```python
from build123d import *

# Parameters (mm, degrees)
SKETCH1_W               = 520
SKETCH1_H               = 75
SKETCH1_W_2             = 440
SKETCH1_H_2             = 60
BOSS_EXTRUDE1_DEPTH     = 10
BOSS_EXTRUDE2_DEPTH     = 575
SKETCH3_W               = 520
SKETCH3_H               = 75
BOSS_EXTRUDE3_DEPTH     = 35
CHAMFER1_SIZE           = 19
CHAMFER1_SIZE_2         = 10.969655115
FILLET1_R               = 30
SKETCH4_R               = 7.5
BOSS_EXTRUDE4_DEPTH     = 20
BOSS_EXTRUDE5_START     = 20
SKETCH5_R               = 7.5
BOSS_EXTRUDE5_DEPTH     = 20
SKETCH6_R               = 15
BOSS_EXTRUDE6_DEPTH     = 30
BOSS_EXTRUDE7_START     = 30
SKETCH7_R               = 15
BOSS_EXTRUDE7_DEPTH     = 30
CUT_EXTRUDE1_DEPTH      = 250
CUT_EXTRUDE1_DEPTH_BACK = 250
SKETCH8_R               = 16.5


with BuildPart() as part:
    # Sketch1 → Boss-Extrude1 (new body)
    with BuildSketch(Plane(origin=(0, 0, 0), x_dir=(0, 0, -1), z_dir=(1, 0, 0))):
        with Locations((0, 37.5)):
            Rectangle(SKETCH1_W, SKETCH1_H)
        with Locations((0, 34)):
            Rectangle(SKETCH1_W_2, SKETCH1_H_2, mode=Mode.SUBTRACT)
    extrude(amount=-BOSS_EXTRUDE1_DEPTH)

    # Sketch2 → Boss-Extrude2 (add)
    with BuildSketch(Plane.ZY.offset(10)):
        Polygon((260, 0), (260, 75), (207, 75), (207, 64), (220, 64), (220, 4), (-220, 4), (-220, 64), (-207, 64), (-207, 75), (-260, 75), (-260, 0), align=None)
    extrude(amount=BOSS_EXTRUDE2_DEPTH)

    # Sketch3 → Boss-Extrude3 (add)
    with BuildSketch(Plane(origin=(0, 0, 0), x_dir=(0, 0, -1), z_dir=(1, 0, 0))):
        with Locations((0, 37.5)):
            Rectangle(SKETCH3_W, SKETCH3_H)
    extrude(amount=BOSS_EXTRUDE3_DEPTH)

    # Chamfer1
    # the kernel refuses this chamfer: 19, 10.969655115 mm, written as the material it takes off along each edge
    with BuildSketch(Plane(origin=(-10, 75, 207), x_dir=(0, 0.01932676561270119, 0.9998132206222079), z_dir=(-1, 0, 0))) as chamfer1_piece_1:
        Polygon((CHAMFER1_SIZE * 0.999813220622, -CHAMFER1_SIZE * 0.0193267656127), (-CHAMFER1_SIZE_2 * 0.019326765612, -CHAMFER1_SIZE_2 * 0.999813220586), (0, 0), align=None)
    extrude(amount=624.154629338, mode=Mode.SUBTRACT)
    with BuildSketch(Plane(origin=(-10, 75, -207), x_dir=(0, 0.057893862402678804, -0.9983227437537922), z_dir=(-1, 0, 0))) as chamfer1_piece_2:
        Polygon((CHAMFER1_SIZE_2 * 0.998322743718, CHAMFER1_SIZE_2 * 0.0578938624006), (-CHAMFER1_SIZE * 0.0578938624027, CHAMFER1_SIZE * 0.998322743754), (0, 0), align=None)
    extrude(amount=624.154629338, mode=Mode.SUBTRACT)

    # Fillet1
    fillet1_edges = [part.edges().sort_by_distance(p)[0] for p in [
        (-585, 75, 243),
        (-585, 75, -238.984827557),
    ]]
    fillet(fillet1_edges, radius=FILLET1_R)

    # Sketch4 → Boss-Extrude4 (add)
    with BuildSketch(Plane.XY.offset(260)):
        with Locations((-568.68, 50)):
            Circle(SKETCH4_R)
    extrude(amount=BOSS_EXTRUDE4_DEPTH)

    # Sketch5 → Boss-Extrude5 (add)
    with BuildSketch(Plane(origin=(0, 0, -260), x_dir=(-1, 0, 0), z_dir=(0, 0, -1)).offset(BOSS_EXTRUDE5_START)):
        with Locations(Location((568.68, 50, 0), (0, 0, 180))):
            Circle(SKETCH5_R)
    extrude(amount=-BOSS_EXTRUDE5_DEPTH)

    # Sketch6 → Boss-Extrude6 (add)
    with BuildSketch(Plane.XY.offset(260)):
        with Locations((10, 35)):
            Circle(SKETCH6_R)
    extrude(amount=BOSS_EXTRUDE6_DEPTH)

    # Sketch7 → Boss-Extrude7 (add)
    with BuildSketch(Plane(origin=(0, 0, -260), x_dir=(-1, 0, 0), z_dir=(0, 0, -1)).offset(BOSS_EXTRUDE7_START)):
        with Locations(Location((-10, 35, 0), (0, 0, 180))):
            Circle(SKETCH7_R)
    extrude(amount=-BOSS_EXTRUDE7_DEPTH)

    # Sketch8 → Cut-Extrude1 (cut, two sides: drawn at the far end of the back side and taken through both)
    with BuildSketch(Plane.XY.offset(-CUT_EXTRUDE1_DEPTH_BACK)):
        with Locations(Location((-25, 35, 0), (0, 0, 180))):
            Circle(SKETCH8_R)
        with Locations(Location((-69, 35, 0), (0, 0, 180))):
            Circle(SKETCH8_R)
        with Locations(Location((-113, 35, 0), (0, 0, 180))):
            Circle(SKETCH8_R)
        with Locations(Location((-157, 35, 0), (0, 0, 180))):
            Circle(SKETCH8_R)
        with Locations(Location((-201, 35, 0), (0, 0, 180))):
            Circle(SKETCH8_R)
        with Locations(Location((-245, 35, 0), (0, 0, 180))):
            Circle(SKETCH8_R)
        with Locations(Location((-289, 35, 0), (0, 0, 180))):
            Circle(SKETCH8_R)
        with Locations(Location((-333, 35, 0), (0, 0, 180))):
            Circle(SKETCH8_R)
        with Locations(Location((-377, 35, 0), (0, 0, 180))):
            Circle(SKETCH8_R)
        with Locations(Location((-421, 35, 0), (0, 0, 180))):
            Circle(SKETCH8_R)
        with Locations(Location((-465, 35, 0), (0, 0, 180))):
            Circle(SKETCH8_R)
        with Locations(Location((-509, 35, 0), (0, 0, 180))):
            Circle(SKETCH8_R)
        with Locations(Location((-553, 35, 0), (0, 0, 180))):
            Circle(SKETCH8_R)
    extrude(amount=CUT_EXTRUDE1_DEPTH + CUT_EXTRUDE1_DEPTH_BACK, mode=Mode.SUBTRACT)


solid = part.part
```
Geometry check sheet. Reference: the model listing, model coordinates, mm. A direction names the side the tool comes from. Give positions to 0.01 mm unless a question says otherwise; leave off trailing zeros. Order: outer loops, then holes, each group sorted by start corner. A loop starts at its lowest first (then second) coordinate and runs counter-clockwise, first axis right, second up. Notation, with made-up numbers: (-10.5, -19.5) - (37.5, -19.5) arc R19 ccw to (37.5, 4.5) - close; hole circle Ø8 at (-7, -5). An arc over 180 degrees is marked (long way). Answer in a Markdown table with one row per item. Add a question column.
Q1. Cross-section at B-B, the plane x = 10. Enter the section's corners in (y, z).
Q2. Mould release check, pull along Z, two halves, no side actions. Record for faces 1 (the cylindrical face through (-392.738, 30.044, -235.21)), 2 (the flat face through (-569, 50, -280)), 3 (the cylindrical face through (-561.526, 52.253, 269.86)): pulls with the +Z half, pulls with the -Z half, needs draft (parallel to the pull), parting line crosses it, or undercut.
Q3. Tool access check on faces 4 (the cylindrical face through (-568.738, 30.044, 234.79)), 5 (the cylindrical face through (18.06, 22.35, -275.21)), 6 (the cylindrical face through (-576.445, 65.979, 239.018)). Record the directions out of +Z, -Z, +X, -X, +Y, -Y that give a thin tool (end or side, any length) a straight path to the whole face; none if there is none.
Q4. Cross-section at A-A, the plane z = -66.5. Enter the section's corners in (x, y), then the cut area to 4 significant figures.
Q5. Gauge pin test, flat ends, axial feed: pin 1 (6 mm diameter, centred on y = 23, z = -186, fed in from -X); pin 2 (20 mm diameter, centred on x = -465, y = 35, fed in from -Z); pin 3 (2 mm diameter, centred on x = -460.5, z = -68, fed in from +Y). Record the tip position at first contact, or that the pin passes through.
Q6. Material ranges on probe 1 along Z at (x, y) = (-329.5, 55.5); probe 2 along Z at (x, y) = (-328, 40.5); probe 3 along Y at (x, z) = (-157, -233), recorded low to high. Write a range as from..to.
Check values:
| question | item | result |
|---|---|---|
| 1 | outline | (0, -260) - (20, -260) - (20, -290) - (50, -290) - (50, -260) - (75, -260) - (75, 260) - (50, 260) - (50, 290) - (20, 290) - (20, 260) - (0, 260) - close |
| 2 | face 1 | undercut |
| 2 | face 2 | pulls with the -Z half |
| 2 | face 3 | needs draft |
| 3 | face 4 | none |
| 3 | face 5 | -Z |
| 3 | face 6 | +Z, -Z, -X, +Y |
| 4 | outline | (-585, 0) - (35, 0) - (35, 75) - (-10, 75) - (-10, 64) - (0, 64) - (0, 4) - (-585, 4) - close |
| 4 | area | 5,075 mm^2 |
| 5 | pin 1 | stops at x = 0 |
| 5 | pin 2 | stops at z = -260 |
| 5 | pin 3 | stops at y = 4 |
| 6 | probe 1 | z = -260..-220, 220..260 |
| 6 | probe 2 | z = -260..-250, 250..260 |
| 6 | probe 3 | y = 0..18.5, 51.5..75 |
